Verification items for the finished model (mm, model axes). A direction names the side the tool comes from. Give positions to 0.01 mm unless a question says otherwise; leave off trailing zeros. Loops run counter-clockwise (first coordinate to the right, second up) from the corner with the lowest first, then second, coordinate; pieces in that order, holes last. Notation, with made-up numbers: M -27.75,-15.75 L 18.25,-15.75 A19 ccw 18.25,18.25 Z; hole C -24.75,32.25 d9. An arc over 180 degrees is marked long. Use a Markdown table: item, result.
from build123d import *

# Parameters (mm, degrees)
PAD_DEPTH               = 10
THICKNESS_T             = 2
SKETCH001_R             = 1
PAD001_DEPTH            = 7.9
SKETCH001_MIRRORED_2_R  = 1
PAD001_MIRRORED_2_DEPTH = 7.9
SKETCH003_W             = 14.25
SKETCH003_H             = 8
POCKET_DEPTH            = 5
FILLET_R                = 1
SKETCH004_W             = 50
SKETCH004_H             = 0.75
SKETCH004_W_2           = 0.75
SKETCH004_H_2           = 25
SKETCH004_H_3           = 13
PAD002_DEPTH            = 1


with BuildPart() as part:
    # Sketch → Pad (new body)
    with BuildSketch(Plane.XY):
        with BuildLine():
            ThreePointArc((-77.75, 37.75), (-81.285534, 36.285534), (-82.75, 32.75))
            Line((-82.75, -32.75), (-82.75, 32.75))
            ThreePointArc((-82.75, -32.75), (-81.285534, -36.285534), (-77.75, -37.75))
            Line((77.75, -37.75), (-77.75, -37.75))
            ThreePointArc((77.75, -37.75), (81.285534, -36.285534), (82.75, -32.75))
            Line((82.75, 32.75), (82.75, -32.75))
            ThreePointArc((82.75, 32.75), (81.285534, 36.285534), (77.75, 37.75))
            Line((-77.75, 37.75), (77.75, 37.75))
        make_face()
    extrude(amount=PAD_DEPTH)

    # Thickness
    thickness_openings = [part.faces().sort_by_distance(p)[0] for p in [
        (0, 0, 10),
    ]]
    offset(amount=THICKNESS_T, openings=thickness_openings, kind=Kind.INTERSECTION)

    # Sketch001 (on Face9 of Thickness) → Pad001 (join)
    with BuildSketch(Plane.XY):
        with BuildLine():
            Line((-77.75, 37.75), (-72.75, 37.75))
            ThreePointArc((-82.75, 27.75), (-75.678932, 30.678932), (-72.75, 37.75))
            Line((-82.75, 32.75), (-82.75, 27.75))
            ThreePointArc((-77.75, 37.75), (-81.285534, 36.285534), (-82.75, 32.75))
        make_face()
        with Locations((-77.5, 32.5)):
            Circle(SKETCH001_R, mode=Mode.SUBTRACT)
    pad001 = extrude(amount=PAD001_DEPTH)

    # Sketch001 Mirrored 2 → Pad001 Mirrored 2 (add)
    with BuildSketch(Plane(origin=(0, 0, 0), x_dir=(-1, 0, 0), z_dir=(0, 0, -1))):
        with BuildLine():
            Line((-77.75, 37.75), (-72.75, 37.75))
            ThreePointArc((-82.75, 27.75), (-75.678932, 30.678932), (-72.75, 37.75))
            Line((-82.75, 32.75), (-82.75, 27.75))
            ThreePointArc((-77.75, 37.75), (-81.285534, 36.285534), (-82.75, 32.75))
        make_face()
        with Locations((-77.5, 32.5)):
            Circle(SKETCH001_MIRRORED_2_R, mode=Mode.SUBTRACT)
    pad001_mirrored_2 = extrude(amount=-PAD001_MIRRORED_2_DEPTH)

    # Mirrored001: Pad001, Pad001 Mirrored 2 across Sketch001 H_Axis
    add(pad001.mirror(Plane.ZX))
    add(pad001_mirrored_2.mirror(Plane.ZX))

    # Sketch003 (on Face19 of MultiTransform) → Pocket (cut)
    with BuildSketch(Plane(origin=(-84.75, 0, 0), x_dir=(0, -1, 0), z_dir=(-1, 0, 0))):
        with Locations((-9.875, 6)):
            Rectangle(SKETCH003_W, SKETCH003_H)
    extrude(amount=-POCKET_DEPTH, mode=Mode.SUBTRACT)

    # Fillet
    fillet_edges = [part.edges().sort_by_distance(p)[0] for p in [
        (0, 39.75, -2),
        (82.699747, 37.699747, -2),
        (84.75, 0, -2),
        (82.699747, -37.699747, -2),
        (0, -39.75, -2),
        (-82.699747, -37.699747, -2),
        (-84.75, 0, -2),
        (-82.699747, 37.699747, -2),
    ]]
    fillet(fillet_edges, radius=FILLET_R)

    # Sketch004 (on Face4 of Fillet) → Pad002 (join)
    with BuildSketch(Plane.XY.offset(10)):
        with Locations((-37.5, 38.125)):
            Rectangle(SKETCH004_W, SKETCH004_H)
        with Locations((37.5, 38.125)):
            Rectangle(SKETCH004_W, SKETCH004_H)
        with Locations((83.125, 0)):
            Rectangle(SKETCH004_W_2, SKETCH004_H_2)
        with Locations((-37.5, -38.125)):
            Rectangle(SKETCH004_W, SKETCH004_H)
        with Locations((37.5, -38.125)):
            Rectangle(SKETCH004_W, SKETCH004_H)
        with Locations((-83.125, -15.25)):
            Rectangle(SKETCH004_W_2, SKETCH004_H_2)
        with Locations((-83.125, 24.9)):
            Rectangle(SKETCH004_W_2, SKETCH004_H_3)
    extrude(amount=PAD002_DEPTH)


solid = part.part
(1) Gauge pin test, flat ends, axial feed: P1, Ø1.6, axis at x = -77.5, y = 32.5, coming from the +Z side; P2, Ø0.8, axis at y = 38, z = 10.5, coming from the +X side; P3, Ø5, axis at x = 77, y = -34, coming from the +Z side; P4, Ø1.1, axis at x = -31, z = 10.5, coming from the -Y side. Record the tip position at first contact, or that the pin passes through.
Results below:
| item | result |
|---|---|
| P1 | z = 0 |
| P2 | x = 62.5 |
| P3 | z = 7.9 |
| P4 | y = -39.75 |
(2) Set-up check for faces 1 (the flat face through (1, -39.75, 4)), 2 (the flat face through (1, -37.75, 5)): record each of +Z, -Z, +X, -X, +Y, -Y from which the full face is reachable in a straight line by a thin tool's end or side.
Results below:
| item | result |
|---|---|
| face 1 | +Z, -Z, +X, -X, -Y |
| face 2 | +Z |
(3) Cross-section at B-B on x = 33.5. Record the cut outline in (y, z).
Results below:
| item | result |
|---|---|
| outline | M -39.75,-1 A1 ccw -38.75,-2 L 38.75,-2 A1 ccw 39.75,-1 L 39.75,10 L 38.5,10 L 38.5,11 L 37.75,11 L 37.75,0 L -37.75,0 L -37.75,11 L -38.5,11 L -38.5,10 L -39.75,10 Z |
(4) Draft check along Y on faces 3 (the flat face through (-79, 34, 7.9)), 4 (the flat face through (-1, 39.75, 4)), 5 (the flat face through (-84.75, 0, 4)). Enter one of: +Y half, -Y half, draft (parallel to the pull), parting line (faces both ways), or undercut.
Results below:
| item | result |
|---|---|
| face 3 | undercut |
| face 4 | +Y half |
| face 5 | draft |
(5) Material ranges on line 1 (Y direction, x = 77.5, z = 3.5); line 2 (Y direction, x = 3, z = 4.75); line 3 (X direction, y = -6, z = 9.5), recorded low to high.
Results below:
| item | result |
|---|---|
| line 1 | -39.75 to -33.5, -31.5 to -29.24, 29.24 to 31.5, 33.5 to 39.75 |
| line 2 | -39.75 to -37.75, 37.75 to 39.75 |
| line 3 | -84.75 to -82.75, 82.75 to 84.75 |
(6) Cross-section at C-C on y = -19.5. Record the cut outline in (x, z).
Results below:
| item | result |
|---|---|
| outline | M -84.75,-1 A1 ccw -83.75,-2 L 83.75,-2 A1 ccw 84.75,-1 L 84.75,10 L 82.75,10 L 82.75,0 L -82.75,0 L -82.75,11 L -83.5,11 L -83.5,10 L -84.75,10 Z |
(7) Cross-section at A-A on z = 5. Record the cut outline in (x, y).
Results below:
| item | result |
|---|---|
| outline | M -84.75,-32.75 A7 ccw -77.75,-39.75 L 77.75,-39.75 A7 ccw 84.75,-32.75 L 84.75,32.75 A7 ccw 77.75,39.75 L -77.75,39.75 A7 ccw -84.75,32.75 L -84.75,17 L -82.75,17 L -82.75,27.75 A10 ccw -72.75,37.75 L 72.75,37.75 A10 ccw 82.75,27.75 L 82.75,-27.75 A10 ccw 72.75,-37.75 L -72.75,-37.75 A10 ccw -82.75,-27.75 L -82.75,2.75 L -84.75,2.75 Z; hole C -77.5,-32.5 d2; hole C -77.5,32.5 d2; hole C 77.5,-32.5 d2; hole C 77.5,32.5 d2 |
